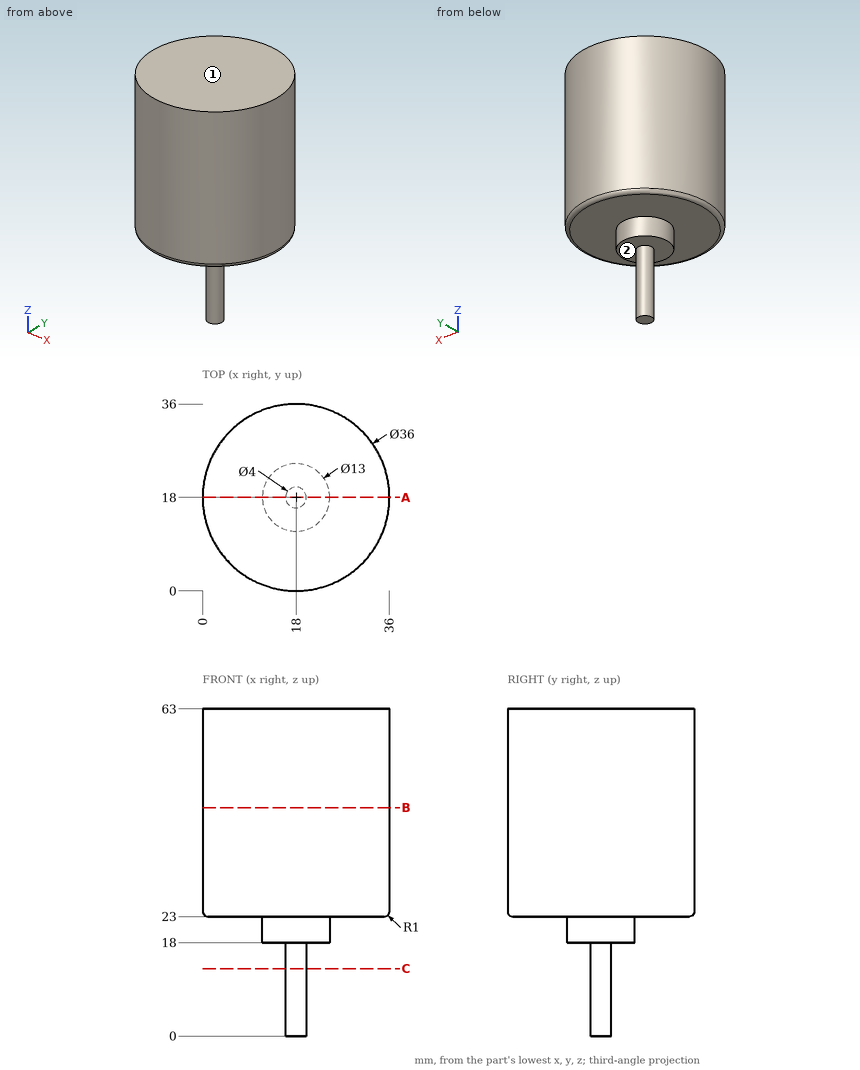
Can you work these out from the drawing? Everything is in mm from the part's minimum corner. A direction names the side the tool comes from. Give positions to 0.01 mm unless a question says otherwise; leave off trailing zeros. Loops run counter-clockwise (first coordinate to the right, second up) from the corner with the lowest first, then second, coordinate; pieces in that order, holes last. Notation, with made-up numbers: (-22, 19.25) - (1, 19.25) arc R26 ccw to (1, 51.25) - close; hole circle Ø11 at (70.5, 47). An arc over 180 degrees is marked (long way). Use one line per item in the form item = value.
1. I want a section at C-C (z = 13). Please give me the cut outline in (x, y), and give its area (3 significant figures).
Response values:
outline = circle Ø4 at (18, 18)
area = 12.6 mm²
2. I need wall thicknesses on probe 1 along Y at (x, z) = (18.5, 50); probe 2 along Z at (x, y) = (9, 9); probe 3 along Z at (x, y) = (18, 24). Which ranges of each line are inside material? Lowest first, please.
Response values:
probe_1 = 0.01 to 35.99
probe_2 = 23 to 63
probe_3 = 18 to 63
3. I'm going to push flat-ended pins straight in: pin 1 Ø4 at (y, z) = (7.5, 34) entering from +X; pin 2 Ø4 at (x, z) = (10, 40) entering from -Y; pin 3 Ø5 at (x, z) = (13.5, 49.5) entering from -Y. Where does each tip first touch, or does it pass through?
Response values:
pin_1 = 33.87
pin_2 = 1.03
pin_3 = 0.11
4. On a 3-axis mill with a long thin cutter (end or side, diameter ignored), from which of +Z, -Z, +X, -X, +Y, -Y can I reach the whole of each face in a straight line? I mean the marked faces 1 and 2. Say none if no direction works.
Response values:
face_1 = +Z, +X, -X, +Y, -Y
face_2 = -Z
5. I want a section at B-B (z = 44). Please give me the cut outline in (x, y).
Response values:
outline = circle Ø36 at (18, 18)
6. I want a section at A-A (y = 18). Please give me the cut outline in (x, z), and give its area (3 significant figures).
Response values:
outline = (0, 24) arc R1 ccw to (1, 23) - (11.5, 23) - (11.5, 18) - (16, 18) - (16, 0) - (20, 0) - (20, 18) - (24.5, 18) - (24.5, 23) - (35, 23) arc R1 ccw to (36, 24) - (36, 63) - (0, 63) - close
area = 1,580 mm²
